from build123d import *

# Parameters (mm, degrees)
PROBEPROFILE_W      = 69.85
PROBEPROFILE_H      = 19.05
PROBEPROFILE_W_2    = 63.5
PROBEPROFILE_H_2    = 12.7
EXTRUDE_THIN1_DEPTH = 25.4
SKETCH2_R           = 15.875
BOSS_EXTRUDE1_DEPTH = 34.925
SKETCH2_2_R         = 15.875
CUT_EXTRUDE1_DEPTH  = 31.75
SKETCH3_W           = 3.175
SKETCH3_H           = 19.05
BOSS_EXTRUDE2_DEPTH = 66.675
CUT_EXTRUDE2_START  = -69.85
SKETCH4_R           = 5.0038
CUT_EXTRUDE2_DEPTH  = 69.85


with BuildPart() as part:
    # ProbeProfile → Extrude-Thin1 (new body)
    with BuildSketch(Plane(origin=(0, 0, 0), x_dir=(1, 0, 0), z_dir=(0, 1, 0))):
        Rectangle(PROBEPROFILE_W, PROBEPROFILE_H)
        Rectangle(PROBEPROFILE_W_2, PROBEPROFILE_H_2, mode=Mode.SUBTRACT)
    extrude(amount=EXTRUDE_THIN1_DEPTH)



with BuildPart() as body_2:
    # Sketch2 → Boss-Extrude1 (new body, symmetric)
    with BuildSketch(Plane(origin=(0, 0, 0), x_dir=(0, 0, -1), z_dir=(1, 0, 0))):
        with Locations((-6.35, -66.675)):
            Circle(SKETCH2_R)
    extrude(amount=BOSS_EXTRUDE1_DEPTH, both=True)

    # Sketch2<2> → Cut-Extrude1 (cut, symmetric)
    with BuildSketch(Plane(origin=(0, 0, 0), x_dir=(0, 0, -1), z_dir=(1, 0, 0))):
        with Locations((-6.35, -66.675)):
            Circle(SKETCH2_2_R)
    extrude(amount=CUT_EXTRUDE1_DEPTH, both=True, mode=Mode.SUBTRACT)


with BuildPart() as part_1:
    add(part.part)

    add(body_2.part)  # Boss-Extrude2 merges body 2
    # Sketch3 → Boss-Extrude2 (add)
    with BuildSketch(Plane.XZ):
        with Locations((33.3375, 0)):
            Rectangle(SKETCH3_W, SKETCH3_H)
        with Locations((-33.3375, 0)):
            Rectangle(SKETCH3_W, SKETCH3_H)
    extrude(amount=BOSS_EXTRUDE2_DEPTH)

    # Sketch4 → Cut-Extrude2 (cut)
    with BuildSketch(Plane.ZY.offset(34.925).offset(CUT_EXTRUDE2_START)):
        with Locations((6.35, -66.675)):
            Circle(SKETCH4_R)
    extrude(amount=CUT_EXTRUDE2_DEPTH, mode=Mode.SUBTRACT)


solid = part_1.part
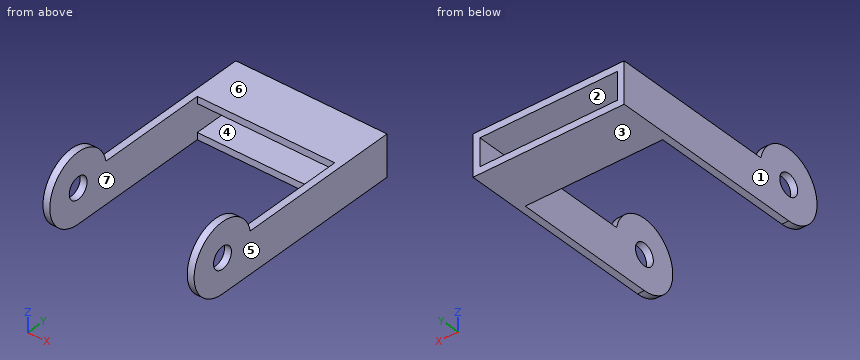
Verification items for the finished model (mm, model axes). Face numbers are marked on the shaded views. A direction names the side the tool comes from. Coordinates: 2 decimals unless noted, no trailing zeros. Order: outer loops, then holes, each group sorted by start corner. A loop starts at its lowest first (then second) coordinate and runs counter-clockwise, first axis right, second up.
Item 1: Section check A-A, the plane y = -45. Enter the section's corners in (x, z) (3 decimals), then the cut area to 3 significant figures.
Filled in:
outline: (-34.925, -9.525) - (-31.75, -9.525) - (-31.75, 9.525) - (-34.925, 9.525) - close; (31.75, -9.525) - (34.925, -9.525) - (34.925, 9.525) - (31.75, 9.525) - close
area: 121 mm2
Item 2: Depth check by flat-ended pin: pin 1 (2.5 mm diameter, centred on x = -10.5, z = -8, fed in from -Y). Enter the tip coordinate at first touch or a pass-through.
Filled in:
pin 1: stops at y = 0
Item 3: Material ranges on L1, parallel to Y at x = -32.7, z = 6.35; L2, parallel to X at y = -31.5, z = -6.5 (3 decimals); L3, parallel to Z at x = 30, y = 1.5 (3 decimals), recorded low to high.
Filled in:
L1: y = -82.55 to -71.68, -61.67 to 25.4
L2: x = -34.925 to -31.75, 31.75 to 34.925
L3: z = -9.525 to -6.35, 6.35 to 9.525
Item 4: Section check B-B, the plane x = -6. Enter the section's corners in (y, z) (3 decimals).
Filled in:
outline: (0, -9.525) - (25.4, -9.525) - (25.4, -6.35) - (0, -6.35) - close; (0, 6.35) - (25.4, 6.35) - (25.4, 9.525) - (0, 9.525) - close
Item 5: Access from +Z, -Z, +X, -X, +Y, -Y to the whole of each face (thin tool, end or side, straight path). Record for the marked faces 4, 5, 6 and 7.
Filled in:
face 4: +Y, -Y
face 5: +Z, -Z, +X, +Y, -Y
face 6: +Z, +X, -X, +Y
face 7: -Y
Item 6: Release check for a two-part mould opening along Z. For the marked faces 1, 2 and 3 record: +Z half, -Z half, draft (parallel to the pull), parting line (faces both ways), or undercut.
Filled in:
face 1: draft
face 2: undercut
face 3: -Z half
